The listing builds one solid part. Answer for the finished solid, in the listing's coordinates (mm). Face numbers are marked on the shaded views. A direction names the side the tool comes from. Give positions to 0.01 mm unless a question says otherwise; leave off trailing zeros. Write each loop counter-clockwise with the first axis right and the second up, starting at its lowest first coordinate (ties: lowest second). Pieces come first, ordered by that corner, then holes. Notation, with made-up numbers: (30.25, 70) -> (73.25, 70) arc R13 ccw to (73.25, 78) -> close; hole circle Ø9 at (41.5, 63). An arc over 180 degrees is marked (long way). Put each result on its own line as item: value. Start each with the question number.
1) Find the intervals of material crossed by line 1 along Y through (x, z) = (-9, 0.7); line 2 along X through (y, z) = (10.5, 1.9); line 3 along X through (y, z) = (-11.5, 0.85) (3 decimals), in increasing order. Write a range as from..to.
2) Flat-ended cylindrical pins translate along their axes: pin 1 Ø2 at (x, z) = (-0.5, 4.5) entering from +Y; pin 2 Ø5 at (x, y) = (0, 0) entering from +Z; pin 3 Ø3 at (x, y) = (-15.5, 2) entering from -Z; pin 4 Ø2 at (x, z) = (11.5, 2.5) entering from -Y. Find the tip coordinate at first contact, or state that the pin passes through.
3) A cutting plane is placed at B-B (y = -14.5). Write down the section's boundary in (x, z).
4) For the marked faces 1 and 2, determine the directions among +Z, -Z, +X, -X, +Y, -Y from which every point of the face is accessible in a straight line to the end or side of a thin tool.
5) A cutting plane is placed at A-A (x = 0). Write down the section's boundary in (y, z).
6) A cutting plane is placed at C-C (x = -13). Write down the section's boundary in (y, z).
7) For a pull along X with two mould halves and no side action, classify the marked faces 3, 4, 5 and 6 as released by +X, released by -X, zero draft, split by the parting line, or undercut.
8) A cutting plane is placed at D-D (z = 2.6). Give the number of separate pieces and of enclosed holes in the cut face, then the cut area to 3 significant figures.
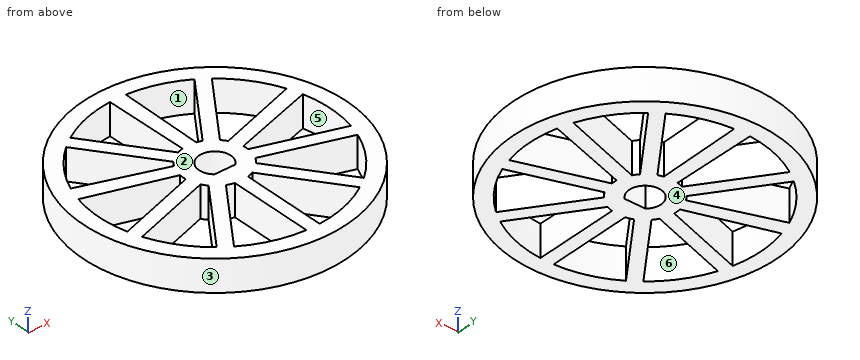
from build123d import *

# Parameters (mm, degrees)
SKETCH1_R           = 25
BOSS_EXTRUDE2_DEPTH = 6


with BuildPart() as part:
    # Sketch1 → Boss-Extrude2 (new body)
    with BuildSketch(Plane.XY):
        Circle(SKETCH1_R)
        with BuildLine():
            Line((-4.534391195, -3.929287021), (-14.005896945, -16.965696295))
            ThreePointArc((-14.005896945, -16.965696295), (-17.85403181, -12.854320212), (-20.532375114, -7.900732383))
            Line((-20.532375114, -7.900732383), (-5.235649328, -2.930524888))
            ThreePointArc((-5.235649328, -2.930524888), (-4.91047904, -3.447781257), (-4.534391195, -3.929287021))
        make_face(mode=Mode.SUBTRACT)
        with BuildLine():
            Line((-2.513596268, -5.448103688), (-11.967457053, -18.460226751))
            ThreePointArc((-11.967457053, -18.460226751), (-6.798373876, -20.923243358), (-1.168772903, -21.968931924))
            Line((-1.168772903, -21.968931924), (-1.168772903, -5.885063288))
            ThreePointArc((-1.168772903, -5.885063288), (-1.854101966, -5.706339098), (-2.513596268, -5.448103688))
        make_face(mode=Mode.SUBTRACT)
        with BuildLine():
            Line((-1.984313483, -2.25), (1.984313483, -2.25))
            ThreePointArc((1.984313483, -2.25), (0, 3), (-1.984313483, -2.25))
        make_face(mode=Mode.SUBTRACT)
        with BuildLine():
            Line((2.513209972, -5.448281898), (11.967106425, -18.460454052))
            ThreePointArc((11.967106425, -18.460454052), (6.888635303, -20.893700095), (1.358822573, -21.957996293))
            Line((1.358822573, -21.957996293), (1.358822573, -5.844108248))
            ThreePointArc((1.358822573, -5.844108248), (1.946106018, -5.675620791), (2.513209972, -5.448281898))
        make_face(mode=Mode.SUBTRACT)
        with BuildLine():
            Line((-21.303090338, -5.493481779), (-5.977939812, -0.514038525))
            ThreePointArc((-5.977939812, -0.514038525), (-5.997955792, 0.156608815), (-5.942969251, 0.825297812))
            Line((-5.942969251, 0.825297812), (-21.282827475, 5.571467909))
            ThreePointArc((-21.282827475, 5.571467909), (-21.999963111, 0.040287778), (-21.303090338, -5.493481779))
        make_face(mode=Mode.SUBTRACT)
        with BuildLine():
            Line((4.534110635, -3.929610763), (14.005574543, -16.965962446))
            ThreePointArc((14.005574543, -16.965962446), (17.888250951, -12.806657562), (20.574373634, -7.790709183))
            Line((20.574373634, -7.790709183), (5.293061004, -2.825509725))
            ThreePointArc((5.293061004, -2.825509725), (4.944500519, -3.398810765), (4.534110635, -3.929610763))
        make_face(mode=Mode.SUBTRACT)
        with BuildLine():
            Line((-11.80762859, 18.562863655), (-2.336164682, 5.526511972))
            ThreePointArc((-2.336164682, 5.526511972), (-1.774817269, 5.731494017), (-1.195863246, 5.879618278))
            Line((-1.195863246, 5.879618278), (-1.395173787, 21.95571657))
            ThreePointArc((-1.395173787, 21.95571657), (-6.815890285, 20.917543824), (-11.80762859, 18.562863655))
        make_face(mode=Mode.SUBTRACT)
        with BuildLine():
            Line((-13.858895862, 17.085988572), (-4.404999409, 4.073816417))
            ThreePointArc((-4.404999409, 4.073816417), (-4.759982517, 3.652747793), (-5.074861212, 3.200903573))
            Line((-5.074861212, 3.200903573), (-20.326913466, 8.415259293))
            ThreePointArc((-20.326913466, 8.415259293), (-17.634136679, 13.154361391), (-13.858895862, 17.085988572))
        make_face(mode=Mode.SUBTRACT)
        with BuildLine():
            Line((13.858571335, 17.0862518), (4.40471055, 4.074128737))
            ThreePointArc((4.40471055, 4.074128737), (4.796457199, 3.604718899), (5.138399164, 3.097878958))
            Line((5.138399164, 3.097878958), (20.46354969, 8.077322211))
            ThreePointArc((20.46354969, 8.077322211), (17.742384309, 13.007989815), (13.858571335, 17.0862518))
        make_face(mode=Mode.SUBTRACT)
        with BuildLine():
            Line((11.807275837, 18.563088032), (2.335770087, 5.526678758))
            ThreePointArc((2.335770087, 5.526678758), (1.862276825, 5.703676448), (1.375565326, 5.840190068))
            Line((1.375565326, 5.840190068), (1.604826213, 21.94138858))
            ThreePointArc((1.604826213, 21.94138858), (6.915515093, 20.884818673), (11.807275837, 18.563088032))
        make_face(mode=Mode.SUBTRACT)
        with BuildLine():
            Line((21.332214938, -5.379275588), (5.987092878, -0.39334319))
            ThreePointArc((5.987092878, -0.39334319), (5.998482577, 0.134932498), (5.963349889, 0.662161691))
            Line((5.963349889, 0.662161691), (21.31722763, 5.438364293))
            ThreePointArc((21.31722763, 5.438364293), (21.999978886, 0.030479888), (21.332214938, -5.379275588))
        make_face(mode=Mode.SUBTRACT)
    extrude(amount=BOSS_EXTRUDE2_DEPTH)


solid = part.part
Reply:
1. line 1: y = -23.32..-20.07, -14.38..-10.08, -4.15..-1.5, 1.77..4.54, 10.4..14.7, 20.07..23.32
1. line 2: x = -22.69..-19.33, -9.07..-5.95, -1.25..1.44, 5.95..9.07, 19.33..22.69
1. line 3: x = -22.198..-18.755, -10.035..-6.911, -1.169..1.359, 6.91..10.034, 18.755..22.198
2. pin 1: stops at y = 25
2. pin 2: stops at z = 6
2. pin 3: passes through
2. pin 4: stops at y = -22.69
3. outline: (-20.37, 0) -> (-16.55, 0) -> (-16.55, 6) -> (-20.37, 6) -> close; (-12.21, 0) -> (-9.09, 0) -> (-9.09, 6) -> (-12.21, 6) -> close; (-1.17, 0) -> (1.36, 0) -> (1.36, 6) -> (-1.17, 6) -> close; (9.09, 0) -> (12.21, 0) -> (12.21, 6) -> (9.09, 6) -> close; (16.55, 0) -> (20.37, 0) -> (20.37, 6) -> (16.55, 6) -> close
4. face 1: +Z, -Z
4. face 2: +Z, +X, -X, +Y, -Y
5. outline: (-25, 0) -> (-2.25, 0) -> (-2.25, 6) -> (-25, 6) -> close; (3, 0) -> (25, 0) -> (25, 6) -> (3, 6) -> close
6. outline: (-21.35, 0) -> (-15.58, 0) -> (-15.58, 6) -> (-21.35, 6) -> close; (-5.45, 0) -> (-2.8, 0) -> (-2.8, 6) -> (-5.45, 6) -> close; (3.01, 0) -> (5.91, 0) -> (5.91, 6) -> (3.01, 6) -> close; (15.9, 0) -> (21.35, 0) -> (21.35, 6) -> (15.9, 6) -> close
7. face 3: split by the parting line
7. face 4: zero draft
7. face 5: undercut
7. face 6: undercut
8. separate pieces: 1
8. enclosed holes: 11
8. area: 945 mm2
